from build123d import *

# Parameters (mm, degrees)
SKETCH1_W           = 25.5443469
SKETCH1_H           = 25.5443469
SKETCH1_W_2         = 21.5443469
SKETCH1_H_2         = 21.5443469
EXTRUDE_THIN1_DEPTH = 21.5443469
SKETCH2_W           = 25.5443469
SKETCH2_H           = 25.5443469
BOSS_EXTRUDE1_DEPTH = 2
BOSS_EXTRUDE2_DEPTH = 2
BOSS_EXTRUDE3_DEPTH = 1
FILLET2_R           = 3
EXTRUDE_THIN2_DEPTH = 2
FILLET3_R           = 1


with BuildPart() as part:
    # Sketch1 → Extrude-Thin1 (new body)
    with BuildSketch(Plane(origin=(0, 0, 0), x_dir=(1, 0, 0), z_dir=(0, 1, 0))):
        with Locations((10.77217345, 10.77217345)):
            Rectangle(SKETCH1_W, SKETCH1_H)
        with Locations((10.77217345, 10.77217345)):
            Rectangle(SKETCH1_W_2, SKETCH1_H_2, mode=Mode.SUBTRACT)
    extrude(amount=EXTRUDE_THIN1_DEPTH)

    # Sketch2 → Boss-Extrude1 (add)
    with BuildSketch(Plane.XZ):
        with Locations((10.77217345, -10.77217345)):
            Rectangle(SKETCH2_W, SKETCH2_H)
    extrude(amount=BOSS_EXTRUDE1_DEPTH)

    # Sketch4 → Boss-Extrude2 (add)
    with BuildSketch(Plane.XZ.offset(2)):
        with BuildLine():
            Line((-0.443258652, 2), (-0.443258652, 17.823551836))
            ThreePointArc((-0.443258652, 17.823551836), (10.77217345, 29.038983939), (21.987605552, 17.823551836))
            Line((21.987605552, 17.823551836), (21.987605552, 2))
            ThreePointArc((21.987605552, 2), (10.77217345, -9.215432102), (-0.443258652, 2))
        make_face()
    extrude(amount=-BOSS_EXTRUDE2_DEPTH)

    # Sketch5 → Boss-Extrude3 (add, symmetric)
    with BuildSketch(Plane(origin=(10.77217345, 0, 0), x_dir=(0, 0, -1), z_dir=(1, 0, 0))):
        Polygon((-2, 9.77217345), (-9.911775918, 0), (-2, 0), align=None)
    extrude(amount=BOSS_EXTRUDE3_DEPTH, both=True)

    # Fillet2
    fillet2_edges = [part.edges().sort_by_distance(p)[0] for p in [
        (9.77217345, 4.886086725, 2),
        (11.77217345, 4.886086725, 2),
    ]]
    fillet(fillet2_edges, radius=FILLET2_R)

    # Sketch6 → Extrude-Thin2 (add)
    with BuildSketch(Plane(origin=(0, 0, 0), x_dir=(1, 0, 0), z_dir=(0, 1, 0))):
        with BuildLine():
            ThreePointArc((-0.443258652, -17.823551836), (10.77217345, -29.038983939), (21.987605552, -17.823551836))
            Line((21.987605552, -17.823551836), (16.987605552, -17.823551836))
            ThreePointArc((16.987605552, -17.823551836), (10.77217345, -24.038983939), (4.556741348, -17.823551836))
            Line((4.556741348, -17.823551836), (-0.443258652, -17.823551836))
        make_face()
    extrude(amount=EXTRUDE_THIN2_DEPTH)

    # Fillet3
    fillet3_edges = [part.edges().sort_by_distance(p)[0] for p in [
        (19.487605552, 0, 17.823551836),
        (2.056741348, 0, 17.823551836),
        (10.77217345, 2, 29.038983939),
        (10.77217345, 2, 24.038983939),
        (10.77217345, 0, 24.038983939),
    ]]
    fillet(fillet3_edges, radius=FILLET3_R - 0.0001)  # a hair under: the kernel refuses the full size


solid = part.part
Design review of the part built by this model. Coordinates are the model's own, in mm. A direction names the side the tool comes from. Round coordinates to 2 decimals unless told otherwise and drop trailing zeros. Write each loop counter-clockwise with the first axis right and the second up, starting at its lowest first coordinate (ties: lowest second). Pieces come first, ordered by that corner, then holes. Notation, with made-up numbers: (73.5, 3) -> (77.5, 3) arc R23 cw to (77.5, 15) -> close; hole circle Ø1 at (65.5, 53). An arc over 180 degrees is marked (long way). One line per item, written item: value. Start each with the question number.
Q1. To check wall thickness, follow probe 1 along Z at (x, y) = (19.5, 20.75); probe 2 along X at (y, z) = (1.5, -11); probe 3 along Z at (x, y) = (4.5, 0.25). State the ranges of each line that lie inside material, in increasing order.
Q2. Add section A-A (y = 7.5). Give the boundary of the cut face in (x, z).
Q3. Tool access review of faces 1 (the face through (11, 11, 0)), 2 (the face through (12.67, 3.87, 2.86)), 3 (the face through (8.87, 3.869, 2.855)), 4 (the face through (-2, 10, -11)), 5 (the face through (11.087, 5.633, 5.351)): name each direction out of +Z, -Z, +X, -X, +Y, -Y from which nothing blocks a thin tool from reaching the whole face with its end or side.
Q4. Add section C-C (y = 12.5). Give the boundary of the cut face in (x, z), then the cut area to 3 significant figures.
Q5. Add section B-B (z = -16.5). Give the boundary of the cut face in (x, y), then the cut area to 3 significant figures.
Q6. The part is to be moulded in two halves that separate along Z. For faces 6 (the face through (19.57, 0.3, 17.54)), 7 (the face through (10.526, -0.521, 29.036)), 8 (the face through (-0.443, -1, 10)), say which applies: pulls with the +Z half, pulls with the -Z half, needs draft (parallel to the pull), parting line crosses it, or undercut.
Q7. Insertion check: P1, Ø10.5, axis at x = 15.5, z = 11, coming from the +Y side; P2, Ø1, axis at x = 20.5, z = 20, coming from the +Y side; P3, Ø1.5, axis at x = 1, y = 15, coming from the +Z side. Each pin has a flat end and moves straight along its axis. Give the tip position at first contact, or say it passes through.
Q8. Add section D-D (z = 6.5). Give the boundary of the cut face in (x, y), then the cut area to 3 significant figures.
Response:
1. probe 1: z = -23.54 to -21.54, 0 to 2
1. probe 2: x = -2 to 0, 21.54 to 23.54
1. probe 3: z = -23.54 to -21.54, 0 to 2, 17.49 to 27.12
2. outline: (-2, -23.54) -> (23.54, -23.54) -> (23.54, 2) -> (14.77, 2) arc R3 cw to (12.01, 3.84) -> (9.54, 3.84) arc R3 cw to (6.77, 2) -> (-2, 2) -> close; hole (0, -21.54) -> (21.54, -21.54) -> (21.54, 0) -> (0, 0) -> close
3. face 1: +Y
3. face 2: +X, +Y
3. face 3: -X, +Y
3. face 4: +Z, -Z, -X, +Y, -Y
3. face 5: +X, -X, +Y
4. outline: (-2, -23.54) -> (23.54, -23.54) -> (23.54, 2) -> (-2, 2) -> close; hole (0, -21.54) -> (21.54, -21.54) -> (21.54, 0) -> (0, 0) -> close
4. area: 188 mm^2
5. outline: (-2, -2) -> (23.54, -2) -> (23.54, 21.54) -> (21.54, 21.54) -> (21.54, 0) -> (0, 0) -> (0, 21.54) -> (-2, 21.54) -> close
5. area: 137 mm^2
6. face 6: undercut
6. face 7: pulls with the +Z half
6. face 8: needs draft
7. P1: stops at y = 3.22
7. P2: stops at y = 2
7. P3: stops at z = 2
8. outline: (-0.44, -2) -> (21.99, -2) -> (21.99, 0) -> (11.77, 0) -> (11.77, 4.21) -> (9.77, 4.21) -> (9.77, 0) -> (-0.44, 0) -> close
8. area: 53.3 mm^2
